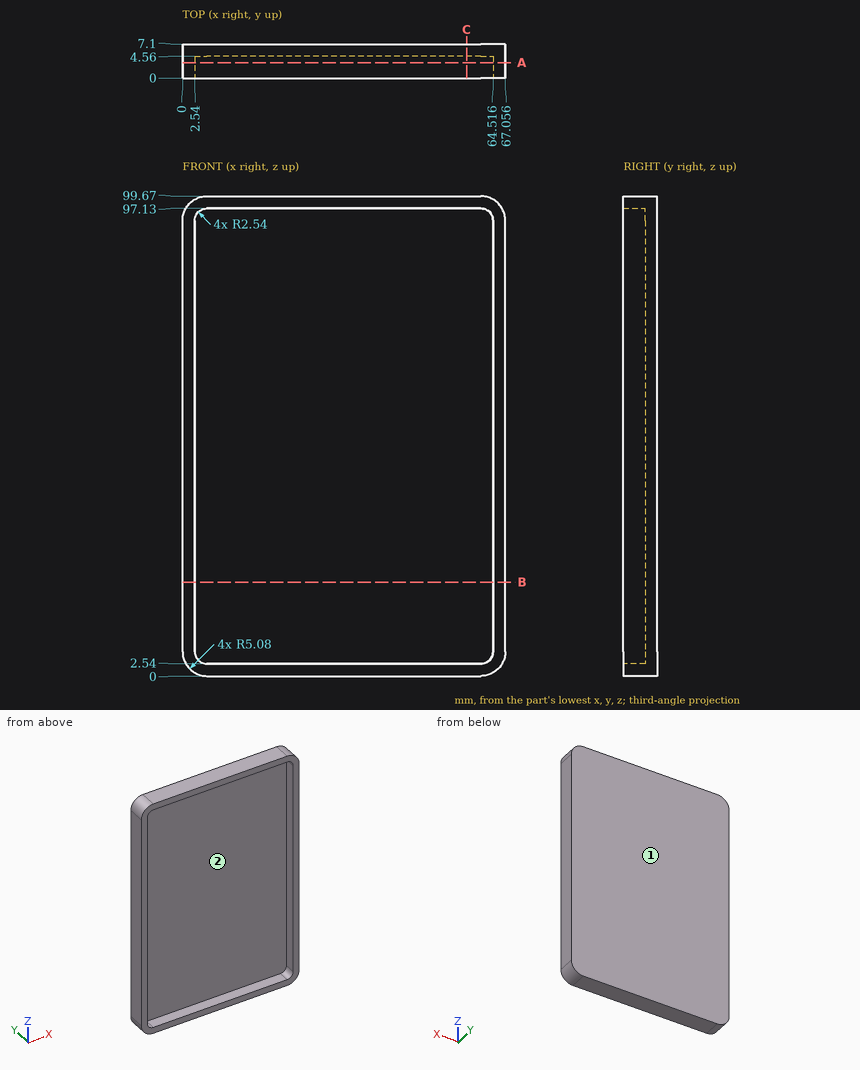
Design review of the part shown in the three views and the two pictorial views. Dimensions are in mm from the part's minimum x, y and z. A direction names the side the tool comes from. Give positions to 0.01 mm unless a question says otherwise; leave off trailing zeros. Write each loop counter-clockwise with the first axis right and the second up, starting at its lowest first coordinate (ties: lowest second). Pieces come first, ordered by that corner, then holes.
Item 1: Take a section at A-A (y = 3.25). Give the boundary of the cut face in (x, z).
Item 2: Take a section at C-C (x = 59). Give the boundary of the cut face in (y, z).
Item 3: Wall thickness on probe 1 along Z at (x, y) = (15, 4.25); probe 2 along X at (y, z) = (1.75, 47); probe 3 along Y at (x, z) = (30, 81.5): over which ranges is each line inside the solid? List them lowest first.
Item 4: Take a section at B-B (z = 19.5). Give the boundary of the cut face in (x, y).
Item 5: Insertion check: P1, Ø4, axis at x = 29.5, z = 63, coming from the -Y side. The pin has a flat end and moves straight along its axis. Give the tip position at first contact, or say it passes through.
Item 6: Machinability: for the marked faces 1 and 2, which of the approach directions +Z, -Z, +X, -X, +Y, -Y give a long, thin tool a straight path to every point of the face, cutting with its end or side? Answer none if there is none.
Established:
1. outline: (0, 5.08) arc R5.08 ccw to (5.08, 0) - (61.98, 0) arc R5.08 ccw to (67.06, 5.08) - (67.06, 94.59) arc R5.08 ccw to (61.98, 99.67) - (5.08, 99.67) arc R5.08 ccw to (0, 94.59) - close; hole (2.54, 5.08) arc R2.54 ccw to (5.08, 2.54) - (61.98, 2.54) arc R2.54 ccw to (64.52, 5.08) - (64.52, 94.59) arc R2.54 ccw to (61.98, 97.13) - (5.08, 97.13) arc R2.54 ccw to (2.54, 94.59) - close
2. outline: (0, 0) - (7.1, 0) - (7.1, 99.67) - (0, 99.67) - (0, 97.13) - (4.56, 97.13) - (4.56, 2.54) - (0, 2.54) - close
3. probe 1: z = 0 to 2.54, 97.13 to 99.67
3. probe 2: x = 0 to 2.54, 64.52 to 67.06
3. probe 3: y = 4.56 to 7.1
4. outline: (0, 0) - (2.54, 0) - (2.54, 4.56) - (64.52, 4.56) - (64.52, 0) - (67.06, 0) - (67.06, 7.1) - (0, 7.1) - close
5. P1: stops at y = 4.56
6. face 1: +Z, -Z, +X, -X, +Y
6. face 2: -Y
